from build123d import *

# Parameters (mm, degrees)
SKETCH1_W               = 150
SKETCH1_H               = 87
BODY_FRAME_DEPTH        = 53
BODY_EDGES_R            = 3
SHELL1_START            = 3
SHELL1_OUTLINE_W        = 81
SHELL1_OUTLINE_H        = 50
SHELL1_DEPTH            = 144
SKETCH3_R               = 1
SCREW_HOLE_DEPTH        = 50
MIRROR2_COPY_1_SKETCH_R = 1
MIRROR2_COPY_1_DEPTH    = 50
SKETCH4_W               = 6
SKETCH4_H               = 5
SKETCH4_R               = 1
BOSS_EXTRUDE3_DEPTH     = 5
SKETCH5_W               = 14
SKETCH5_H               = 9
SWITCH_DEPTH            = 179.849098404
SKETCH6_W               = 28
SKETCH6_H               = 20
AC_IN_DEPTH             = 3
SKETCH8_W               = 8
SKETCH8_H               = 13
PROGRAM_PORT_DEPTH      = 3
CUT_EXTRUDE1_DEPTH      = 182.322916367
LPATTERN1_COUNT         = 5
LPATTERN1_PITCH         = 12


# Read off the part's stored shape, not the designer's step: Shell1
with BuildPart() as part:
    # Sketch1 → Body_frame (new body)
    with BuildSketch(Plane.XY):
        with Locations((75, 43.5)):
            Rectangle(SKETCH1_W, SKETCH1_H)
    extrude(amount=BODY_FRAME_DEPTH)

    # body_edges
    body_edges_edges = [part.edges().sort_by_distance(p)[0] for p in [
        (0, 87, 26.5),
        (150, 87, 26.5),
        (150, 0, 26.5),
        (0, 0, 26.5),
    ]]
    fillet(body_edges_edges, radius=BODY_EDGES_R)

    # Shell1 outline → Shell1 (cut)
    with BuildSketch(Plane.YZ.offset(SHELL1_START)):
        with Locations((43.5, 28)):
            Rectangle(SHELL1_OUTLINE_W, SHELL1_OUTLINE_H)
    extrude(amount=SHELL1_DEPTH, mode=Mode.SUBTRACT)

    # Sketch3 → screw_hole (add)
    with BuildSketch(Plane.XY.offset(3)):
        with BuildLine():
            Line((3, 84), (8, 84))
            Line((8, 84), (8, 81.5))
            ThreePointArc((8, 81.5), (7.267766953, 79.732233047), (5.5, 79))
            Line((5.5, 79), (3, 79))
            Line((3, 79), (3, 84))
        make_face()
        with Locations((5.5, 81.5)):
            Circle(SKETCH3_R, mode=Mode.SUBTRACT)
    screw_hole = extrude(amount=SCREW_HOLE_DEPTH)

    # Mirror1: screw_hole across plane
    add(screw_hole.mirror(Plane.ZY.offset(-75)))

    # Mirror2: screw_hole across plane
    add(screw_hole.mirror(Plane.ZX.offset(43.5)))

    # Mirror2 copy 1 sketch → Mirror2 copy 1 (add)
    with BuildSketch(Plane(origin=(150, 87, 3), x_dir=(-1, 0, 0), z_dir=(0, 0, 1))):
        with BuildLine():
            Line((3, 84), (8, 84))
            Line((8, 84), (8, 81.5))
            ThreePointArc((8, 81.5), (7.267766953, 79.732233047), (5.5, 79))
            Line((5.5, 79), (3, 79))
            Line((3, 79), (3, 84))
        make_face()
        with Locations((5.5, 81.5)):
            Circle(MIRROR2_COPY_1_SKETCH_R, mode=Mode.SUBTRACT)
    extrude(amount=MIRROR2_COPY_1_DEPTH)

    # Sketch4 → Boss-Extrude3 (add)
    # profile 1 of 4: a face of its own
    with BuildSketch(Plane.XY.offset(3)):
        with Locations((6, 76.5)):
            Rectangle(SKETCH4_W, SKETCH4_H)
        with Locations((6, 76.5)):
            Circle(SKETCH4_R, mode=Mode.SUBTRACT)
    # profile 2 of 4: a face of its own
    with BuildSketch(Plane.XY.offset(3)):
        with Locations((90, 76.5)):
            Rectangle(SKETCH4_W, SKETCH4_H)
        with Locations((90, 76.5)):
            Circle(SKETCH4_R, mode=Mode.SUBTRACT)
    # profile 3 of 4: a face of its own
    with BuildSketch(Plane.XY.offset(3)):
        with Locations((6, 26.5)):
            Rectangle(SKETCH4_W, SKETCH4_H)
        with Locations((6, 26.5)):
            Circle(SKETCH4_R, mode=Mode.SUBTRACT)
    # profile 4 of 4: a face of its own
    with BuildSketch(Plane.XY.offset(3)):
        with Locations((90, 26.5)):
            Rectangle(SKETCH4_W, SKETCH4_H)
        with Locations((90, 26.5)):
            Circle(SKETCH4_R, mode=Mode.SUBTRACT)
    extrude(amount=BOSS_EXTRUDE3_DEPTH)

    # Sketch5 → switch (cut, through all)
    with BuildSketch(Plane(origin=(3, 0, 0), x_dir=(0, 0, -1), z_dir=(1, 0, 0))):
        with Locations((-13, 16)):
            Rectangle(SKETCH5_W, SKETCH5_H)
    extrude(amount=-SWITCH_DEPTH, mode=Mode.SUBTRACT)

    # Sketch6 → AC_IN (cut)
    with BuildSketch(Plane.XZ):
        with Locations((123.5, 35)):
            Rectangle(SKETCH6_W, SKETCH6_H)
    extrude(amount=-AC_IN_DEPTH, mode=Mode.SUBTRACT)

    # Sketch8 → Program_port (cut)
    with BuildSketch(Plane.ZY):
        with Locations((18.5, 64)):
            Rectangle(SKETCH8_W, SKETCH8_H)
    extrude(amount=-PROGRAM_PORT_DEPTH, mode=Mode.SUBTRACT)

    # Sketch9 → Cut-Extrude1 (cut, through all)
    with BuildSketch(Plane.XZ):
        Polygon((18, 18), (23, 18), (34.547005384, 38), (29.547005384, 38), align=None)
    cut_extrude1 = extrude(amount=-CUT_EXTRUDE1_DEPTH, mode=Mode.SUBTRACT)

    # LPattern1: Cut-Extrude1 ×5
    with Locations(*[(i * LPATTERN1_PITCH, 0, 0) for i in range(1, LPATTERN1_COUNT)]):
        add(cut_extrude1, mode=Mode.SUBTRACT)


solid = part.part
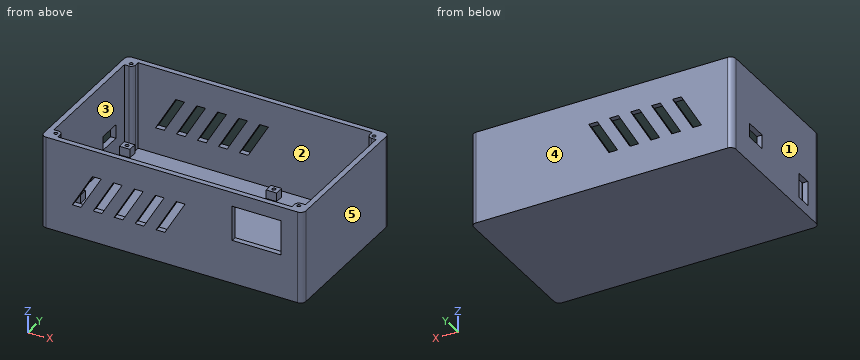
The listing builds one solid part. Answer for the finished solid, in the listing's coordinates (mm). Face numbers are marked on the shaded views. A direction names the side the tool comes from. Coordinates: 2 decimals unless noted, no trailing zeros. Order: outer loops, then holes, each group sorted by start corner. A loop starts at its lowest first (then second) coordinate and runs counter-clockwise, first axis right, second up.
Q1. For a pull along Y with two mould halves and no side action, classify the marked faces 3, 4 and 5 as pulls with the +Y half, pulls with the -Y half, needs draft (parallel to the pull), parting line crosses it, or undercut.
Q2. Which of the six approach directions +Z, -Z, +X, -X, +Y, -Y give full straight-line access (tool end or side, diameter ignored) to the marked faces 1 and 2?
Q3. A cutting plane is placed at A-A, the plane z = 41.5. State how many separate pieces and enclosed holes the cut face has, and give its area (3 significant figures).
Q4. A cutting plane is placed at B-B, the plane y = 72. Write down the section's boundary in (x, z), and give its area (3 significant figures).
Q5. A cutting plane is placed at C-C, the plane x = 38. Write down the section's boundary in (y, z).
Q6. A cutting plane is placed at D-D, the plane y = 14.5. Write down the section's boundary in (x, z), and give its area (3 significant figures).
Q7. Consider line 1 (X direction, y = 5.5, z = 23); line 2 (Y direction, x = 24.5, z = 12.5); line 3 (X direction, y = 24, z = 8.5). Determine where each line is inside the solid, lowest interval first.
Q8. Given P1, Ø4, axis at x = 68.5, y = 12.5, coming from the -Z side; P2, Ø2, axis at x = 98.5, y = 77.5, coming from the +Z side; P3, Ø1.5, axis at x = 91, y = 26, coming from the +Z side, each flat-ended and moving along its own axis, determine where each tip first touches the part or whether it passes through.
Answers follow:
1. face 3: undercut
1. face 4: pulls with the +Y half
1. face 5: needs draft
2. face 1: +Z, -Z, -X, +Y, -Y
2. face 2: +Z
3. separate pieces: 1
3. enclosed holes: 4
3. area: 1,380 mm2
4. outline: (0, 0) - (150, 0) - (150, 53) - (147, 53) - (147, 3) - (3, 3) - (3, 53) - (0, 53) - close
4. area: 750 mm2
5. outline: (0, 0) - (87, 0) - (87, 23.2) - (84, 23.2) - (84, 3) - (3, 3) - (3, 23.2) - (0, 23.2) - close; (0, 31.86) - (3, 31.86) - (3, 53) - (0, 53) - close; (84, 31.86) - (87, 31.86) - (87, 53) - (84, 53) - close
6. outline: (0, 0) - (150, 0) - (150, 53) - (147, 53) - (147, 3) - (3, 3) - (3, 6) - (0, 6) - close; (0, 20) - (3, 20) - (3, 53) - (0, 53) - close
6. area: 708 mm2
7. line 1: x = 0 to 4.5, 6.5 to 8, 142 to 143.5, 145.5 to 150
7. line 2: y = 0 to 3, 84 to 87
7. line 3: x = 0 to 3, 147 to 150
8. P1: stops at z = 0
8. P2: stops at z = 3
8. P3: stops at z = 8
